```python
from build123d import *

# Parameters (mm, degrees)
F1_DEPTH  = 12.954
F3_D      = 27.94
F3_DEPTH  = 20.32
F5_DEPTH  = 25.4
F8_DEPTH  = 34.919414
F9_R      = 8.513263
F10_DEPTH = 117.073686


with BuildPart() as f1:
    # F0 (on Top) → F1 (new body)
    with BuildSketch(Plane.XY):
        with BuildLine():
            Line((70.253901, 21.234231), (70.253901, 21.401851))
            Line((70.253901, 21.401851), (-70.253901, 21.401851))
            Line((-70.253901, 21.401851), (-70.253901, 21.418785))
            ThreePointArc((-70.253901, 21.418785), (-91.672686, 0), (-70.253901, -21.418785))
            Line((-70.253901, -21.418785), (-70.253901, -21.401851))
            Line((-70.253901, -21.401851), (70.253901, -21.401851))
            Line((70.253901, -21.401851), (70.253901, -21.234231))
            ThreePointArc((70.253901, -21.234231), (91.488132, 0), (70.253901, 21.234231))
        make_face()
    extrude(amount=F1_DEPTH)

    # F3
    with Locations(Plane(origin=(0, 0, 0), x_dir=(1, 0, 0), z_dir=(0, 0, -1))):
        with Locations((-65.522589, 0), (66.181116, 0)):
            Hole(F3_D / 2, depth=F3_DEPTH)

    # F4 (on Right) → F5 (join)
    with BuildSketch(Plane.YZ):
        with BuildLine():
            Line((-13.499629, 7.572964), (13.499629, 7.572964))
            Line((13.499629, 7.572964), (13.499629, 43.132961))
            ThreePointArc((13.499629, 43.132961), (0, 56.63259), (-13.499629, 43.132961))
            Line((-13.499629, 43.132961), (-13.499629, 7.572964))
        make_face()
    extrude(amount=F5_DEPTH)

    # F6: F1 across face


with BuildPart() as f1_1:
    add(f1.part)
    add(f1.part.mirror(Plane(origin=(0, 0, 33.456079), x_dir=(0, 1, 0), z_dir=(-1, 0, 0))))

    # F7 (on face) → F8 (cut, through all)
    with BuildSketch(Plane.XZ.offset(13.499629)):
        Polygon((-10.16, 59.448242), (-10.16, 43.132961), (-10.16, 34.201402), (10.16, 34.201402), (10.16, 43.132961), (10.16, 59.448242), align=None)
        with BuildLine():
            Line((10.16, 34.201402), (-10.16, 34.201402))
            ThreePointArc((-10.16, 34.201402), (0, 24.041402), (10.16, 34.201402))
        make_face()
    extrude(amount=-F8_DEPTH, mode=Mode.SUBTRACT)

    # F9 (on face) → F10 (cut, through all)
    with BuildSketch(Plane(origin=(-25.4, 0, 0), x_dir=(0, -1, 0), z_dir=(-1, 0, 0))):
        with Locations((0, 43.132961)):
            Circle(F9_R)
    extrude(amount=-F10_DEPTH, mode=Mode.SUBTRACT)


solid = f1_1.part
```
Geometry check sheet. Reference: the model listing, model coordinates, mm. A direction names the side the tool comes from. Give positions to 0.01 mm unless a question says otherwise; leave off trailing zeros. Order: outer loops, then holes, each group sorted by start corner. A loop starts at its lowest first (then second) coordinate and runs counter-clockwise, first axis right, second up.
1. Section check C-C, the plane z = 48.5. Enter the section's corners in (x, y), and give its area (3 significant figures).
2. Section check B-B, the plane y = 0. Enter the section's corners in (x, z).
3. Access from +Z, -Z, +X, -X, +Y, -Y to the whole of each face (thin tool, end or side, straight path). Record for faces 1 (the face through (-25.4, 0, 30)), 2 (the face through (25.4, 0, 30)), 3 (the face through (0, -13.5, 22)), 4 (the face through (79.49, 0.3, 6.57)), 5 (the face through (10.16, 0, 53)).
4. Gauge pin test, flat ends, axial feed: pin 1 Ø15 at (x, z) = (4.5, 30.5) entering from -Y; pin 2 Ø10 at (y, z) = (2, 32) entering from -X; pin 3 Ø14 at (x, z) = (4, 6.5) entering from +Y. Record the tip position at first contact, or that the pin passes through.
5. Thickness scan on L1, parallel to Z at x = -21.5, y = 0; L2, parallel to X at y = 13, z = 37; L3, parallel to Y at x = -10.5, z = 19. Record the ranges inside material, lowest first.
6. Section check D-D, the plane x = -73.5. Enter the section's corners in (y, z), and give its area (3 significant figures).
7. Section check A-A, the plane x = 13. Enter the section's corners in (y, z), and give its area (3 significant figures).
Values follow:
1. outline: (-25.4, -12.39) - (-10.16, -12.39) - (-10.16, -6.61) - (-25.4, -6.61) - close; (-25.4, 6.61) - (-10.16, 6.61) - (-10.16, 12.39) - (-25.4, 12.39) - close; (10.16, -12.39) - (25.4, -12.39) - (25.4, -6.61) - (10.16, -6.61) - close; (10.16, 6.61) - (25.4, 6.61) - (25.4, 12.39) - (10.16, 12.39) - close
1. area: 352 mm2
2. outline: (-91.67, 0) - (-79.49, 0) - (-79.49, 12.95) - (-91.67, 12.95) - close; (-52.21, 0) - (52.21, 0) - (52.21, 12.95) - (25.4, 12.95) - (25.4, 34.62) - (10.16, 34.62) - (10.16, 34.2) arc R10.16 cw to (-10.16, 34.2) - (-10.16, 34.62) - (-25.4, 34.62) - (-25.4, 12.95) - (-52.21, 12.95) - close; (-25.4, 51.65) - (-10.16, 51.65) - (-10.16, 56.63) - (-25.4, 56.63) - close; (10.16, 51.65) - (25.4, 51.65) - (25.4, 56.63) - (10.16, 56.63) - close; (79.49, 0) - (91.67, 0) - (91.67, 12.95) - (79.49, 12.95) - close
3. face 1: +Z, -X, +Y, -Y
3. face 2: +Z, +X, +Y, -Y
3. face 3: +Z, +X, -X, -Y
3. face 4: +Z, -Z
3. face 5: +Z, +Y, -Y
4. pin 1: stops at y = -13.5
4. pin 2: stops at x = -25.4
4. pin 3: stops at y = 21.4
5. L1: z = 0 to 34.62, 51.65 to 56.63
5. L2: x = -25.4 to -10.16, 10.16 to 25.4
5. L3: y = -13.5 to 13.5
6. outline: (-21.17, 0) - (-11.47, 0) - (-11.47, 12.95) - (-21.17, 12.95) - close; (11.47, 0) - (21.17, 0) - (21.17, 12.95) - (11.47, 12.95) - close
6. area: 251 mm2
7. outline: (-21.4, 0) - (21.4, 0) - (21.4, 12.95) - (13.5, 12.95) - (13.5, 43.13) arc R13.5 ccw to (-13.5, 43.13) - (-13.5, 12.95) - (-21.4, 12.95) - close; hole circle Ø17.03 at (0, 43.13)
7. area: 1,430 mm2
